Can you work these out from the model? Positions are in its coordinate system, mm. A direction names the side the tool comes from. Coordinates: 2 decimals unless noted, no trailing zeros. Order: outer loops, then holes, each group sorted by start corner. A loop starts at its lowest first (then second) coordinate and runs counter-clockwise, first axis right, second up. Notation, with made-up numbers: (-22.75, 56) - (-4.75, 56) arc R35 cw to (-4.75, 91) - close; hole circle Ø6 at (31, -19.75). An arc over 180 degrees is marked (long way). Return JSON: item names as keys, results as strings. Group by question number.
1) Imagine slicing it at D-D (x = 11). Write out the boundary of the cut face in (y, z) (3 decimals).
2) If I drill on line 1 along Z through (x, y) = (30, 25); line 2 along Z through (x, y) = (-30.5, 11.5); line 3 along Z through (x, y) = (28.5, 19.5), over which ranges is the centre line in solid material (lowest first)?
3) Imagine slicing it at A-A (x = -46.5). Write out the boundary of the cut face in (y, z).
4) For pin 1 Ø1 at (x, z) = (-31.5, -43) entering from +Y (3 decimals); pin 2 Ø5 at (y, z) = (8, -29.5) entering from -X; pin 3 Ø12 at (y, z) = (23.5, -26.5) entering from -X; pin 4 Ø19 at (x, z) = (8, -28) entering from +Y, each with a flat end and sliding along its axis, tell me the tip position at first contact or that it passes through.
5) Which directions (+Z, -Z, +X, -X, +Y, -Y) give clear straight access to the entire face, cutting with the end or side of a thin tool? Please do faces 1 (the face through (3, 26.4, 0)), 2 (the face through (-20, 4.175, 25)), 3 (the face through (39.105, -0.014, 9.783)).
6) If we mould it in two halves opening along Z, with no side actions, what happens to faces 4 (the face through (-9, -1, -1)), 5 (the face through (30.191, -0.014, 45.344)), 6 (the face through (-10, 4.175, -13))? For each: pulls with the +Z half, pulls with the -Z half, needs draft (parallel to the pull), parting line crosses it, or undercut.
7) Imagine slicing it at B-B (z = -16). Write out the boundary of the cut face in (x, y) (3 decimals), and give its area (3 significant figures).
8) Imagine slicing it at C-C (y = 22.25). Give the number of separate pieces and of enclosed holes in the cut face, and give its area (3 significant figures).
```python
from build123d import *

# Parameters (mm, degrees)
BOSS_EXTRUDE1_DEPTH = 1
BOSS_EXTRUDE2_DEPTH = 25.4
SKETCH4_R           = 14.351
CUT_EXTRUDE1_DEPTH  = 25.4
SKETCH4_4_R         = 19.177
CUT_EXTRUDE2_DEPTH  = 22.225
LPATTERN1_COUNT     = 3
LPATTERN1_PITCH     = 78
SPLIT3_START        = -1
SPLIT3_DEPTH        = 27.4


# Read off the part's stored shape, not the designer's step: Split3
with BuildPart() as part:
    # Sketch1 → Boss-Extrude1 (new, symmetric)
    with BuildSketch(Plane(origin=(0, 0, 0), x_dir=(1, 0, 0), z_dir=(0, 1, 0))):
        Polygon((118, 0), (-118, 0), (-118, -67.135), (118, -75), align=None)
        Polygon((-118, 67.135), (-118, 0), (118, 0), (118, 75), align=None)
    extrude(amount=BOSS_EXTRUDE1_DEPTH, both=True)

    # Sketch3 → Boss-Extrude2 (add)
    with BuildSketch(Plane(origin=(0, 1, 0), x_dir=(1, 0, 0), z_dir=(0, 1, 0))):
        Polygon((-84.001477372, 20.6375), (-73.002954744, 39.6875), (-84.001477372, 58.7375), (-105.998522628, 58.7375), (-116.997045256, 39.6875), (-105.998522628, 20.6375), align=None)
        Polygon((-38.632571531, 19.84375), (-49.631094159, 0.79375), (-71.628139415, 0.79375), (-82.626662043, 19.84375), (-71.628139415, 38.89375), (-49.631094159, 38.89375), align=None)
        Polygon((-84.001477372, -19.05), (-73.002954744, 0), (-84.001477372, 19.05), (-105.998522628, 19.05), (-116.997045256, 0), (-105.998522628, -19.05), align=None)
        Polygon((-105.998522628, -58.7375), (-84.001477372, -58.7375), (-73.002954744, -39.6875), (-84.001477372, -20.6375), (-105.998522628, -20.6375), (-116.997045256, -39.6875), align=None)
        Polygon((-71.628139415, -38.89375), (-49.631094159, -38.89375), (-38.632571531, -19.84375), (-49.631094159, -0.79375), (-71.628139415, -0.79375), (-82.626662043, -19.84375), align=None)
    boss_extrude2 = extrude(amount=BOSS_EXTRUDE2_DEPTH)

    # Sketch4 → Cut-Extrude1 (cut)
    with BuildSketch(Plane(origin=(0, 26.4, 0), x_dir=(1, 0, 0), z_dir=(0, 1, 0))):
        with Locations(Location((-95, 0, 0), (0, 0, 270))):
            Circle(SKETCH4_R)
        with Locations(Location((-95, -39.6875, 0), (0, 0, 270))):
            Circle(SKETCH4_R)
        with Locations(Location((-95, 39.6875, 0), (0, 0, 90))):
            Circle(SKETCH4_R)
        with Locations(Location((-60.629616787, 19.84375, 0), (0, 0, 270))):
            Circle(SKETCH4_R)
        with Locations(Location((-60.629616787, -19.84375, 0), (0, 0, 90))):
            Circle(SKETCH4_R)
    cut_extrude1 = extrude(amount=-CUT_EXTRUDE1_DEPTH, mode=Mode.SUBTRACT)

    # Sketch4<4> → Cut-Extrude2 (cut)
    with BuildSketch(Plane(origin=(0, 26.4, 0), x_dir=(1, 0, 0), z_dir=(0, 1, 0))):
        with Locations((-95, 0)):
            Circle(SKETCH4_4_R)
        with Locations((-95, -39.6875)):
            Circle(SKETCH4_4_R)
        with Locations((-95, 39.6875)):
            Circle(SKETCH4_4_R)
        with Locations((-60.629616787, 19.84375)):
            Circle(SKETCH4_4_R)
        with Locations((-60.629616787, -19.84375)):
            Circle(SKETCH4_4_R)
    cut_extrude2 = extrude(amount=-CUT_EXTRUDE2_DEPTH, mode=Mode.SUBTRACT)

    # LPattern1: Boss-Extrude2, Cut-Extrude1, Cut-Extrude2 ×3
    with Locations(*[(i * LPATTERN1_PITCH, 0, 0) for i in range(1, LPATTERN1_COUNT)]):
        add(boss_extrude2)
        add(cut_extrude1, mode=Mode.SUBTRACT)
        add(cut_extrude2, mode=Mode.SUBTRACT)

    # Split3 outline → Split3 (cut)
    with BuildSketch(Plane(origin=(0, 0, 0), x_dir=(1, 0, 0), z_dir=(0, 1, 0)).offset(SPLIT3_START)):
        Polygon((33.456794404, 0), (44.913588808, -19.84375), (15.04996756, -71.5690593), (118, -75), (118, 75), (15.04996756, 71.5690593), (44.913588808, 19.84375), align=None)
        Polygon((-118, -67.135), (-61.477571296, -69.018681787), (-33.086411192, -19.84375), (-44.543205596, 0), (-33.086411192, 19.84375), (-61.477571296, 69.018681787), (-118, 67.135), align=None)
    extrude(amount=SPLIT3_DEPTH, mode=Mode.SUBTRACT)


solid = part.part
```
Calculated:
{
 "1": {"outline": "(-1, -71.434) - (1, -71.434) - (1, -38.894) - (26.4, -38.894) - (26.4, -37.932) - (4.175, -37.932) - (4.175, -32.703) - (1, -32.703) - (1, -6.984) - (4.175, -6.984) - (4.175, -1.756) - (26.4, -1.756) - (26.4, -0.794) - (1, -0.794) - (1, 0.794) - (26.4, 0.794) - (26.4, 1.756) - (4.175, 1.756) - (4.175, 6.984) - (1, 6.984) - (1, 32.703) - (4.175, 32.703) - (4.175, 37.932) - (26.4, 37.932) - (26.4, 38.894) - (1, 38.894) - (1, 71.434) - (-1, 71.434) - close"},
 "2": {"line 1": "-36.07 to -34.27, -5.41 to -3.62, 3.62 to 5.41, 34.27 to 36.07", "line 2": "-54.4 to -53.31, -26.07 to -24.97, -14.72 to -13.62, 13.62 to 14.72, 24.97 to 26.07, 53.31 to 54.4", "line 3": "-38.67 to -35.46, -4.23 to -1.02, 1.02 to 4.23, 35.46 to 38.67"},
 "3": {"outline": "(-1, -69.52) - (1, -69.52) - (1, -43.08) - (-1, -43.08) - close; (-1, 43.08) - (1, 43.08) - (1, 69.52) - (-1, 69.52) - close"},
 "4": {"pin 1": "y = 4.175", "pin 2": "x = -32.4", "pin 3": "x = -34.85", "pin 4": "y = 26.4"},
 "5": {"face 1": "+Z, -Z, +X, -X, +Y", "face 2": "+Y", "face 3": "+X, +Y, -Y"},
 "6": {"face 4": "needs draft", "face 5": "pulls with the +Z half", "face 6": "undercut"},
 "7": {"outline": "(-35.306, -1) - (42.694, -1) - (42.694, 1) - (37.148, 1) - (37.148, 26.4) - (36.158, 26.4) - (36.158, 4.175) - (31.197, 4.175) - (31.197, 1) - (3.544, 1) - (3.544, 4.175) - (-1.417, 4.175) - (-1.417, 26.4) - (-2.407, 26.4) - (-2.407, 1) - (-4.241, 1) - (-4.241, 26.4) - (-6.428, 26.4) - (-6.428, 4.175) - (-27.572, 4.175) - (-27.572, 26.4) - (-29.759, 26.4) - (-29.759, 1) - (-35.306, 1) - close", "area": "416 mm2"},
 "8": {"separate pieces": "30", "enclosed holes": "0", "area": "520 mm2"}
}
